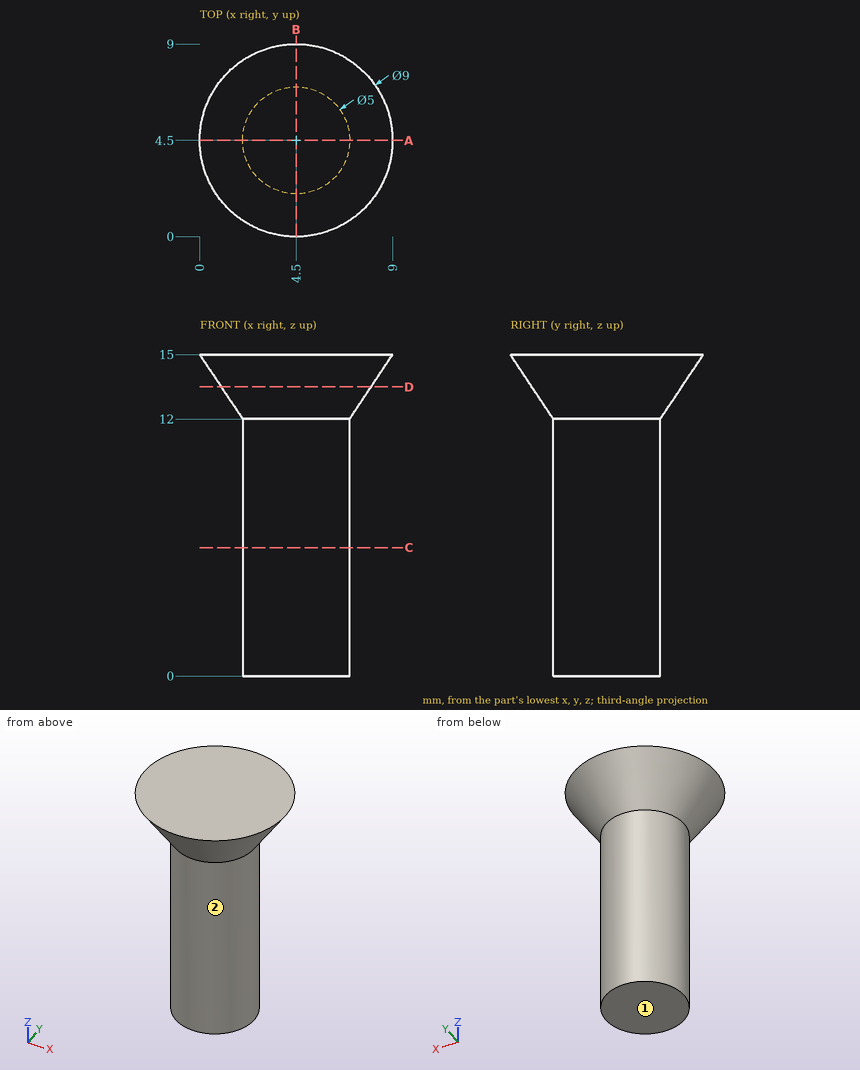
Geometry: see drawing. Coordinates: mm, zero at the bounding-box minimum. A direction names the side the tool comes from. Round coordinates to 2 decimals unless told otherwise and drop trailing zeros. Order: outer loops, then holes, each group sorted by start corner. A loop starts at its lowest first (then second) coordinate and runs counter-clockwise, first axis right, second up. Notation, with made-up numbers: (76.5, 39) - (86.5, 39) arc R14 ccw to (86.5, 54) - close; hole circle Ø5 at (5.5, -21.75). An arc over 180 degrees is marked (long way). Use a Markdown table: item, result. Add a question column.
1. Section query D-D (z = 13.5). Return the cut outline in (x, y).
2. Section query A-A (y = 4.5). Return the cut outline in (x, z).
3. Line query: probe 1 along Y at (x, z) = (4.75, 6); probe 2 along Y at (x, z) = (2.5, 12.75); probe 3 along X at (y, z) = (6.5, 11.5). Output: solid intervals per line, ascending.
4. Set-up query: the marked faces 1 and 2. Return all of +Z, -Z, +X, -X, +Y, -Y with unobstructed straight access to the full face (end or side cutting, diameter ignored); none if empty.
5. Section query C-C (z = 6). Return the cut outline in (x, y).
6. First-contact query: pin 1 (4 mm diameter, centred on x = 6.5, z = 7.5, fed in from -Y); pin 2 (3 mm diameter, centred on y = 6, z = 5.5, fed in from +X); pin 3 (1 mm diameter, centred on y = 2.5, z = 11.5, fed in from -X). Flat tips, straight axial feed; report the tip coordinate or a pass-through.
Derived:
| question | item | result |
|---|---|---|
| 1 | outline | circle Ø7 at (4.5, 4.5) |
| 2 | outline | (0, 15) - (2, 12) - (2, 0) - (7, 0) - (7, 12) - (9, 15) - close |
| 3 | probe 1 | 2.01 to 6.99 |
| 3 | probe 2 | 2.26 to 6.74 |
| 3 | probe 3 | 3 to 6 |
| 4 | face 1 | -Z, +X, -X, +Y, -Y |
| 4 | face 2 | -Z |
| 5 | outline | circle Ø5 at (4.5, 4.5) |
| 6 | pin 1 | y = 2 |
| 6 | pin 2 | x = 7 |
| 6 | pin 3 | x = 2.5 |
